The figure shows three views and two pictorial views of one solid part (mm, origin at its lowest corner). Answer the questions. A direction names the side the tool comes from. Coordinates: 2 decimals unless noted, no trailing zeros. Write each loop counter-clockwise with the first axis right and the second up, starting at its lowest first coordinate (ties: lowest second). Pieces come first, ordered by that corner, then holes.
Item 1: Section B-B (z = 13.5) is taken. Give the vertices of the cut face in (x, y).
Item 2: Section C-C (x = 10) is taken. Give the vertices of the cut face in (y, z).
Item 3: Section A-A (y = 5) is taken. State how many separate pieces and enclosed holes the cut face has, then the cut area to 3 significant figures.
Item 4: Each of these flat-tipped pins is pushed along its axis until it touches: P1, Ø2.5, axis at x = 10, y = 3.5, coming from the +Z side; P2, Ø3.5, axis at x = 22.5, y = 5, coming from the +Z side; P3, Ø3, axis at x = 12, y = 2.5, coming from the +Z side; P4, Ø8.5, axis at x = 31.5, z = 43.5, coming from the -Y side. Where does it stop, or does it pass through?
Item 5: A tool of negligible diameter and unlimited length cuts with its end or side. For the marked faces 4, 5 and 6, from which of +Z, -Z, +X, -X, +Y, -Y can it reach the whole face along a straight path? Write none if from no direction.
Item 6: Section D-D (z = 45.5) is taken. Give the vertices of the cut face in (x, y) (1 decimal).
Item 7: Straight lines are drawn through the part: probe 1 along X at (y, z) = (4.25, 36.5); probe 2 along X at (y, z) = (5.25, 57) (1 decimal); probe 3 along Z at (x, y) = (27, 0.5) (1 decimal). For each, find the intervals that lie inside material, in ascending order.
Item 8: Determine the mould class of the marked faces 1, 2 and 3 for opening direction Z: released by +Z, released by -Z, zero draft, split by the parting line, or undercut.
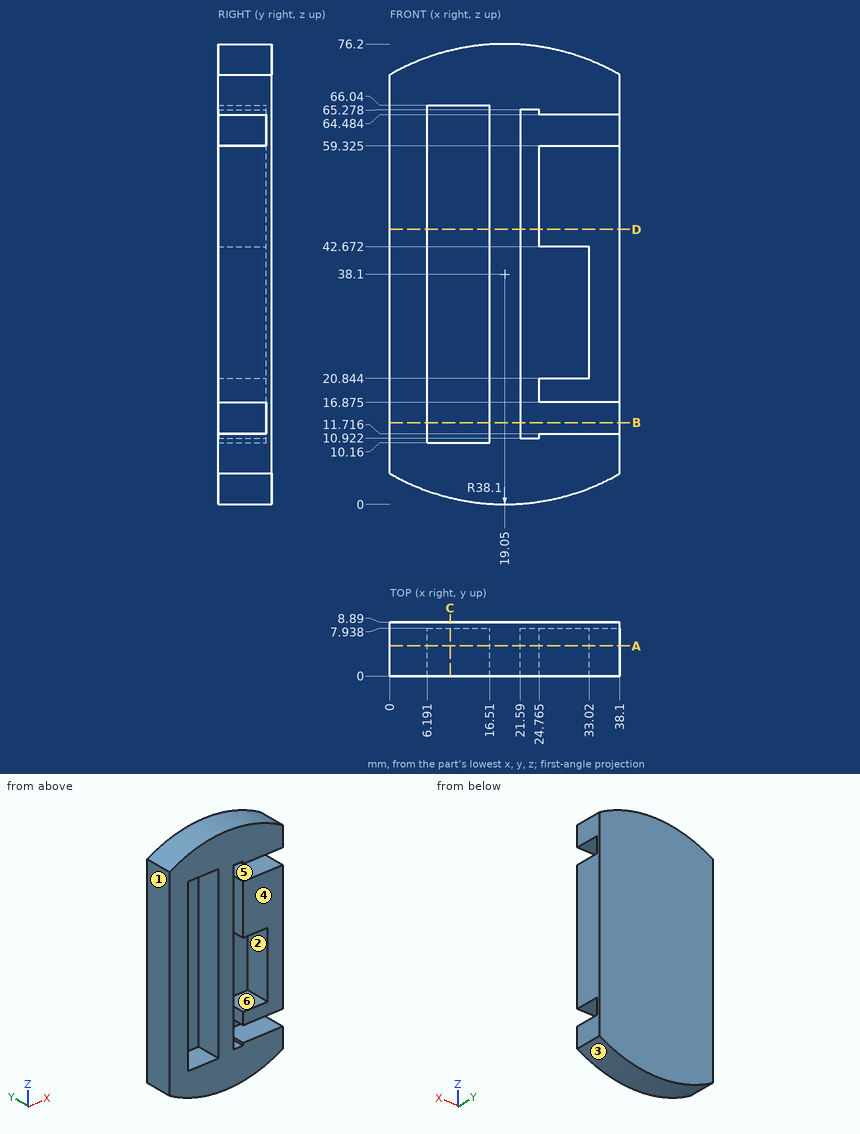
Established:
1. outline: (0, 0) - (6.19, 0) - (6.19, 7.94) - (16.51, 7.94) - (16.51, 0) - (21.59, 0) - (21.59, 7.94) - (38.1, 7.94) - (38.1, 8.89) - (0, 8.89) - close
2. outline: (0, 1.09) - (8.89, 1.09) - (8.89, 75.11) - (0, 75.11) - (0, 66.04) - (7.94, 66.04) - (7.94, 10.16) - (0, 10.16) - close
3. separate pieces: 2
3. enclosed holes: 1
3. area: 1,710 mm2
4. P1: stops at z = 75.39
4. P2: stops at z = 76.16
4. P3: stops at z = 75.79
4. P4: stops at y = 0
5. face 4: +Z, -Z, +X, -X, -Y
5. face 5: +X, -Y
5. face 6: -Y
6. outline: (0, 0) - (6.2, 0) - (6.2, 7.9) - (16.5, 7.9) - (16.5, 0) - (21.6, 0) - (21.6, 7.9) - (24.8, 7.9) - (24.8, 0) - (38.1, 0) - (38.1, 8.9) - (0, 8.9) - close
7. probe 1: x = 0 to 6.19, 16.51 to 21.59, 33.02 to 38.1
7. probe 2: x = 0 to 6.2, 16.5 to 21.6, 24.8 to 38.1
7. probe 3: z = 0.8 to 11.7, 16.9 to 20.8, 42.7 to 59.3, 64.5 to 75.4
8. face 1: zero draft
8. face 2: undercut
8. face 3: released by -Z
